The model under review builds one solid part; all positions refer to its coordinate system, in mm. A direction names the side the tool comes from. Coordinates: 2 decimals unless noted, no trailing zeros. Write each loop counter-clockwise with the first axis right and the second up, starting at its lowest first coordinate (ties: lowest second). Pieces come first, ordered by that corner, then holes.
```python
from build123d import *

# Parameters (mm, degrees)
F1_DEPTH = 15
F2_R     = 2.125
F3_DEPTH = 25
F4_R     = 2.125
F5_DEPTH = 25
F7_DEPTH = 10
F9_DEPTH = 10


with BuildPart() as f1:
    # F0 (on Front) → F1 (new body)
    with BuildSketch(Plane.XZ):
        Polygon((5, 50), (0, 50), (0, 0), (50, 0), (50, 5), (35, 5), (5, 35), align=None)
    extrude(amount=F1_DEPTH)

    # F2 (on face) → F3 (cut)
    with BuildSketch(Plane.XY.offset(5)):
        with Locations((42.5, -7.5)):
            Circle(F2_R)
    extrude(amount=-F3_DEPTH, mode=Mode.SUBTRACT)

    # F4 (on face) → F5 (cut)
    with BuildSketch(Plane.YZ.offset(5)):
        with Locations((-7.5, 42.5)):
            Circle(F4_R)
    extrude(amount=-F5_DEPTH, mode=Mode.SUBTRACT)

    # F6 (on face) → F7 (cut)
    with BuildSketch(Plane.XZ.offset(15)):
        Polygon((35, 5), (5, 35), (5, 15), (15, 5), align=None)
    extrude(amount=-F7_DEPTH, mode=Mode.SUBTRACT)

    # F8 (on face) → F9 (cut)
    with BuildSketch(Plane.XZ.offset(15)):
        Polygon((7.928932, 5), (5, 7.928932), (5, 5), align=None)
    extrude(amount=-F9_DEPTH, mode=Mode.SUBTRACT)


solid = f1.part
```
Item 1: To check wall thickness, follow line 1 along Z through (x, y) = (2.25, -7.5) (3 decimals); line 2 along Y through (x, z) = (42.5, 2.5) (3 decimals); line 3 along X through (y, z) = (-8.25, 23.5). State the ranges of each line that lie inside material, in increasing order.
Solved:
line 1: z = 0 to 40.375, 44.625 to 50
line 2: y = -15 to -9.625, -5.375 to 0
line 3: x = 0 to 5
Item 2: Mouldability with a two-part tool opening along Z and no side actions: class faces 3 (the face through (25, -7, 0)), 4 (the face through (0, -7, 25)), 5 (the face through (6, -5, 6)) as pulls with the +Z half, pulls with the -Z half, needs draft (parallel to the pull), parting line crosses it, or undercut.
Solved:
face 3: pulls with the -Z half
face 4: needs draft
face 5: undercut
Item 3: For pin 1 (5 mm diameter, centred on y = -7.5, z = 42.5, fed in from +X); pin 2 (9 mm diameter, centred on x = 13.5, z = 16, fed in from -Y); pin 3 (8 mm diameter, centred on x = 21.5, y = -9.5, fed in from +Z), all flat-tipped, find the tip position at first contact; note any pin that passes through.
Solved:
pin 1: stops at x = 5
pin 2: stops at y = -5
pin 3: stops at z = 5
Item 4: Take a section at A-A, the plane y = -7.5. Write out the cut boundary in (x, z) (3 decimals).
Solved:
outline: (0, 0) - (40.375, 0) - (40.375, 5) - (15, 5) - (5, 15) - (5, 40.375) - (0, 40.375) - close; (0, 44.625) - (5, 44.625) - (5, 50) - (0, 50) - close; (44.625, 0) - (50, 0) - (50, 5) - (44.625, 5) - close; hole (5, 5) - (7.929, 5) - (5, 7.929) - close
Item 5: Take a section at D-D, the plane y = -13.75. Write out the cut boundary in (x, z), plus the area to 3 significant figures.
Solved:
outline: (0, 0) - (50, 0) - (50, 5) - (15, 5) - (5, 15) - (5, 50) - (0, 50) - close; hole (5, 5) - (7.93, 5) - (5, 7.93) - close
area: 521 mm2
Item 6: Machinability: for faces 1 (the face through (2.535, -6.519, 40.615)), 2 (the face through (5, -9, 32)), which of the approach directions +Z, -Z, +X, -X, +Y, -Y give a long, thin tool a straight path to every point of the face, cutting with its end or side? Answer none if there is none.
Solved:
face 1: +X, -X
face 2: +Z, +X, -Y
Item 7: Take a section at C-C, the plane z = 42.5. Write out the cut boundary in (x, y) (3 decimals), plus the area to 4 significant figures.
Solved:
outline: (0, -15) - (5, -15) - (5, -9.625) - (0, -9.625) - close; (0, -5.375) - (5, -5.375) - (5, 0) - (0, 0) - close
area: 53.75 mm2
Item 8: Take a section at B-B, the plane x = 3. Write out the cut boundary in (y, z) (3 decimals).
Solved:
outline: (-15, 0) - (0, 0) - (0, 50) - (-15, 50) - close; hole circle Ø4.25 at (-7.5, 42.5)
